Autodesk Inventor part; units mm, degrees
ref_plane "YZ Plane" through (0, 0, 0) normal (1, 0, 0) x (0, 1, 0)
ref_plane "XZ Plane" through (0, 0, 0) normal (0, 1, 0) x (-1, 0, 0)
ref_plane "XY Plane" through (0, 0, 0) normal (0, 0, 1) x (1, 0, 0)
sketch "Sketch1" plane through (0, 0, 0) normal (0, 0, 1) x (1, 0, 0)
  line L0 (0, 0) -> (33.25, 0)
  line L1 (33.25, 0) -> (33.25, 33.25)
  line L2 (33.25, 33.25) -> (0, 33.25)
  line L3 (0, 33.25) -> (0, 0)
  dimension "d0" = 33.25
  dimension "d1" = 33.25
extrude "Extrusion1" add sketch "Sketch1" along normal blind 30
sketch "Sketch2" plane through (0, 0, 30) normal (0, 0, 1) x (1, 0, 0)
  point P0 (0, 0)
sketch "Sketch3" plane through (0, 0, 30) normal (0, 0, 1) x (1, 0, 0)
  line L0 (3.25, 3.25) -> (30, 3.25)
  line L1 (30, 3.25) -> (30, 30)
  line L2 (30, 30) -> (3.25, 30)
  line L3 (3.25, 30) -> (3.25, 3.25)
  line L4 (33.25, 0) -> (33.25, 33.25)
  line L5 (0, 0) -> (33.25, 0)
  line L6 (33.25, 0) -> (33.25, 33.25)
  line L7 (33.25, 33.25) -> (0, 33.25)
  line L8 (0, 33.25) -> (0, 0)
  dimension "d4" = 26.75
  dimension "d5" = 26.75
extrude "Extrusion2" cut sketch "Sketch3" against normal blind 26.75 contours L3 L2 L1 L0
chamfer "Chamfer1" distance 1.875 angle 45 8 edges at (33.25, 33.25, 15) (33.25, 0, 15) (0, 33.25, 15) (0, 0, 15) (0, 16.625, 0) (16.625, 33.25, 0) (16.625, 0, 0) (33.25, 16.625, 0)
sketch "Sketch4" plane through (0, 0, 0) normal (0, 0, -1) x (-1, 0, 0)
  circle A0 centre (-16.625, 16.625) radius 4.625
  point P0 (0, 0)
  dimension "d11" = 9.25
extrude "Extrusion3" cut sketch "Sketch4" against normal blind 10
thread "Thread1"
properties part number "cuvette holder lid_with_threaded_escape_valve"
Verification items for the finished model (mm, model axes). A direction names the side the tool comes from. Give positions to 0.01 mm unless a question says otherwise; leave off trailing zeros. Write each loop counter-clockwise with the first axis right and the second up, starting at its lowest first coordinate (ties: lowest second). Pieces come first, ordered by that corner, then holes. Notation, with made-up numbers: (38.5, -10.75) -> (51.5, -10.75) arc R29 ccw to (51.5, 17.25) -> close; hole circle Ø2 at (59, 8.5). An arc over 180 degrees is marked (long way). Use CSV: the item, a comma, the result in double quotes.
(1) Release check for a two-part mould opening along X. For faces 1 (the flat face through (17, 33.25, 16)), 2 (the flat face through (17, 30, 17)), 3 (the flat face through (1.28, 1.31, 1.16)) record: +X half, -X half, draft (parallel to the pull), parting line (faces both ways), or undercut.
Derived:
face 1,"draft"
face 2,"undercut"
face 3,"-X half"
(2) Sectioned sample at B-B (x = 6). Record the cut outline in (y, z) (3 decimals).
Derived:
outline,"(0, 1.875) -> (1.875, 0) -> (31.375, 0) -> (33.25, 1.875) -> (33.25, 30) -> (30, 30) -> (30, 3.25) -> (3.25, 3.25) -> (3.25, 30) -> (0, 30) -> close"
(3) Set-up check for faces 4 (the flat face through (1.28, 31.94, 1.16)), 5 (the flat face through (3.25, 17, 17)): record each of +Z, -Z, +X, -X, +Y, -Y from which the full face is reachable in a straight line by a thin tool's end or side.
Derived:
face 4,"-Z, -X, +Y"
face 5,"+Z"
(4) Go/stop test with flat-tipped pins: pin 1 (6 mm diameter, centred on x = 25, y = 28.5, fed in from +Z); pin 2 (15 mm diameter, centred on x = 16.625, y = 16.625, fed in from +Z). Record where each tip stops, or that it passes through.
Derived:
pin 1,"stops at z = 30"
pin 2,"stops at z = 3.25"
(5) Sectioned sample at A-A (z = 14.75). Record the cut outline in (x, y) (3 decimals), plus the area to 3 significant figures.
Derived:
outline,"(0, 1.875) -> (1.875, 0) -> (31.375, 0) -> (33.25, 1.875) -> (33.25, 31.375) -> (31.375, 33.25) -> (1.875, 33.25) -> (0, 31.375) -> close; hole (3.25, 3.25) -> (30, 3.25) -> (30, 30) -> (3.25, 30) -> close"
area,"383 mm^2"
(6) Material ranges on L1, parallel to Y at x = 9.5, z = 6.5; L2, parallel to Z at x = 6, y = 26, recorded low to high.
Derived:
L1,"y = 0 to 3.25, 30 to 33.25"
L2,"z = 0 to 3.25"
